```python
from build123d import *

# Parameters (mm, degrees)
SKETCH1_W               = 60
SKETCH1_H               = 30
BOSS_EXTRUDE1_DEPTH     = 35
CUT_EXTRUDE1_DEPTH      = 49.476798574
CUT_EXTRUDE1_DEPTH_BACK = 49.476798574
SKETCH3_W               = 6.5
SKETCH3_H               = 10.55
CUT_EXTRUDE2_DEPTH      = 72.063352018
CUT_EXTRUDE2_DEPTH_BACK = 72.063352018
SKETCH4_R               = 6


with BuildPart() as part:
    # Sketch1 → Boss-Extrude1 (new, symmetric)
    with BuildSketch(Plane.XY):
        Rectangle(SKETCH1_W, SKETCH1_H)
    extrude(amount=BOSS_EXTRUDE1_DEPTH, both=True)

    # Sketch3 → Cut-Extrude1 (cut, two sides: drawn at the far end of the back side and taken through both)
    with BuildSketch(Plane.XY.offset(-CUT_EXTRUDE1_DEPTH_BACK)):
        with Locations((15, 9.725)):
            Rectangle(SKETCH3_W, SKETCH3_H)
        with Locations((-15, 9.725)):
            Rectangle(SKETCH3_W, SKETCH3_H)
        with Locations((-15, -9.725)):
            Rectangle(SKETCH3_W, SKETCH3_H)
        with Locations((15, -9.725)):
            Rectangle(SKETCH3_W, SKETCH3_H)
    extrude(amount=CUT_EXTRUDE1_DEPTH + CUT_EXTRUDE1_DEPTH_BACK, mode=Mode.SUBTRACT)

    # Sketch4 → Cut-Extrude2 (cut, two sides: drawn at the far end of the back side and taken through both)
    with BuildSketch(Plane.ZY.offset(30).offset(-CUT_EXTRUDE2_DEPTH_BACK)):
        Circle(SKETCH4_R)
    extrude(amount=CUT_EXTRUDE2_DEPTH + CUT_EXTRUDE2_DEPTH_BACK, mode=Mode.SUBTRACT)


solid = part.part
```
Geometry: final body of the model. Coordinates: model frame, mm. A direction names the side the tool comes from. Coordinates: 2 decimals unless noted, no trailing zeros. Order: outer loops, then holes, each group sorted by start corner. A loop starts at its lowest first (then second) coordinate and runs counter-clockwise, first axis right, second up. Notation, with made-up numbers: (-9, 84) - (43, 84) arc R32 ccw to (43, 117) - close; hole circle Ø2 at (62, 42). An arc over 180 degrees is marked (long way). Write each question's results on one line, items separated by ' | '.
(1) Section query D-D, the plane y = 0. Return the cut outline in (x, z), plus the area to 3 significant figures.
Values found:
outline: (-30, -35) - (30, -35) - (30, -6) - (-30, -6) - close; (-30, 6) - (30, 6) - (30, 35) - (-30, 35) - close | area: 3,480 mm²
(2) Set-up query: faces 1 (the face through (18.25, -10, 0)), 2 (the face through (0, 15, 0)), 3 (the face through (-15, 4.45, 19)). Return all of +Z, -Z, +X, -X, +Y, -Y with unobstructed straight access to the full face (end or side cutting, diameter ignored); none if empty.
Values found:
face 1: +Z, -Z, -Y | face 2: +Z, -Z, +X, -X, +Y | face 3: +Z, -Z, +Y
(3) Mould query, pull axis X, two halves, no side actions, for faces 4 (the face through (24, 15, 0)), 5 (the face through (11.75, -10, 0)). Classes: +X half, -X half, draft (parallel to the pull), parting line (faces both ways), or undercut.
Values found:
face 4: draft | face 5: undercut
(4) Section query C-C, the plane y = 7.5. Return the cut outline in (x, z).
Values found:
outline: (-30, -35) - (-18.25, -35) - (-18.25, 35) - (-30, 35) - close; (-11.75, -35) - (11.75, -35) - (11.75, 35) - (-11.75, 35) - close; (18.25, -35) - (30, -35) - (30, 35) - (18.25, 35) - close
(5) Section query B-B, the plane z = 0. Return the cut outline in (x, y), plus the area to 3 significant figures.
Values found:
outline: (-30, -15) - (-18.25, -15) - (-18.25, -6) - (-30, -6) - close; (-30, 6) - (-18.25, 6) - (-18.25, 15) - (-30, 15) - close; (-11.75, -15) - (11.75, -15) - (11.75, -6) - (-11.75, -6) - close; (-11.75, 6) - (11.75, 6) - (11.75, 15) - (-11.75, 15) - close; (18.25, -15) - (30, -15) - (30, -6) - (18.25, -6) - close; (18.25, 6) - (30, 6) - (30, 15) - (18.25, 15) - close | area: 846 mm²
(6) Section query A-A, the plane x = -15. Return the cut outline in (y, z).
Values found:
outline: (-4.45, -35) - (4.45, -35) - (4.45, -4.02) arc R6 cw to (-4.45, -4.02) - close; (-4.45, 4.02) arc R6 cw to (4.45, 4.02) - (4.45, 35) - (-4.45, 35) - close
(7) First-contact query: pin 1 Ø5 at (x, z) = (-15.5, -26) entering from +Y; pin 2 Ø3 at (x, z) = (14, 25) entering from -Y. Flat tips, straight axial feed; report the tip coordinate or a pass-through.
Values found:
pin 1: stops at y = 4.45 | pin 2: stops at y = -4.45
(8) Line query: line 1 (X direction, y = -11.25, z = -8); line 2 (Z direction, x = -16.5, y = 0); line 3 (Z direction, x = -23, y = -1). Output: solid intervals per line, ascending. Write a range as [from, to].
Values found:
line 1: x = [-30, -18.25], [-11.75, 11.75], [18.25, 30] | line 2: z = [-35, -6], [6, 35] | line 3: z = [-35, -5.92], [5.92, 35]
